Can you work these out from the model? Positions are in its coordinate system, mm. A direction names the side the tool comes from. Round coordinates to 2 decimals unless told otherwise and drop trailing zeros. Order: outer loops, then holes, each group sorted by start corner. A loop starts at its lowest first (then second) coordinate and runs counter-clockwise, first axis right, second up.
Q1. If we section it at D-D (y = 6.5): Please give me the cut outline in (x, z), plus the area to 3 significant figures.
Q2. If we section it at B-B (z = -5): Please give me the cut outline in (x, y).
Q3. We'd pull the mould along X, two halves only. Please class faces 1 (the face through (134.287, 1.662, 2.229)), 2 (the face through (1.713, 62.338, 2.229)), 3 (the face through (67, 32, 0)), 4 (the face through (67, 32, 2.5)): pulls with the +X half, pulls with the -X half, needs draft (parallel to the pull), parting line crosses it, or undercut.
Q4. For faces 5 (the face through (69.846, 53.951, -6.409)), 6 (the face through (1.662, 1.713, 2.229)), which set-ups out of +Z, -Z, +X, -X, +Y, -Y let a thin tool reach every point of the face, with its end or its side?
Q5. If we section it at A-A (x = 129.5): Please give me the cut outline in (y, z), plus the area to 3 significant figures.
Q6. If we section it at C-C (y = 57.5): Please give me the cut outline in (x, z), plus the area to 3 significant figures.
Q7. If I drill on line 1 (X direction, y = 57, z = -6.25); line 2 (X direction, y = 55, z = -8.5); line 3 (Z direction, x = 61, y = 21.5), over which ranges is the centre line in solid material (lowest first)?
Q8. Will these pins go through, and if not, where does the flat tip stop? P1, Ø1.5, axis at x = 71.5, y = 47.5, coming from the -Z side; P2, Ø1.5, axis at x = 36, z = -1, coming from the +Y side; P3, Ø4, axis at y = 12.5, z = -1, coming from the -X side.
from build123d import *

# Parameters (mm, degrees)
PAD_DEPTH       = 2.5
SKETCH002_R     = 4
PAD001_DEPTH    = 15
CHAMFER_SIZE    = 1
CHAMFER001_SIZE = 2


with BuildPart() as part:
    # Sketch → Pad (new body)
    with BuildSketch(Plane.XY):
        with BuildLine():
            Line((4, 0), (132, 0))
            ThreePointArc((132, 0), (134.828427, 1.171573), (136, 4))
            Line((136, 4), (136, 60))
            ThreePointArc((136, 60), (134.828427, 62.828427), (132, 64))
            Line((132, 64), (4, 64))
            ThreePointArc((4, 64), (1.171573, 62.828427), (0, 60))
            Line((0, 60), (0, 4))
            ThreePointArc((0, 4), (1.171573, 1.171573), (4, 0))
        make_face()
    extrude(amount=PAD_DEPTH)

    # Sketch002 → Pad001 (join)
    with BuildSketch(Plane.XY):
        with Locations((6.5, 6.5)):
            Circle(SKETCH002_R)
        with Locations((129.5, 6.5)):
            Circle(SKETCH002_R)
        with Locations((129.5, 57.5)):
            Circle(SKETCH002_R)
        with Locations((6.5, 57.5)):
            Circle(SKETCH002_R)
        with Locations((68, 57.5)):
            Circle(SKETCH002_R)
    extrude(amount=-PAD001_DEPTH)

    # Chamfer
    chamfer_edges = [part.edges().sort_by_distance(p)[0] for p in [
        (68, 0, 2.5),
        (134.828427, 1.171573, 2.5),
        (136, 32, 2.5),
        (134.828427, 62.828427, 2.5),
        (68, 64, 2.5),
        (1.171573, 62.828427, 2.5),
        (0, 32, 2.5),
        (1.171573, 1.171573, 2.5),
    ]]
    chamfer(chamfer_edges, length=CHAMFER_SIZE)

    # Chamfer001
    chamfer001_edges = [part.edges().sort_by_distance(p)[0] for p in [
        (2.5, 6.5, -15),
        (2.5, 57.5, -15),
        (64, 57.5, -15),
        (125.5, 57.5, -15),
        (125.5, 6.5, -15),
    ]]
    chamfer(chamfer001_edges, length=CHAMFER001_SIZE)


solid = part.part
Solution:
1. outline: (0, 0) - (2.5, 0) - (2.5, -13) - (4.5, -15) - (8.5, -15) - (10.5, -13) - (10.5, 0) - (125.5, 0) - (125.5, -13) - (127.5, -15) - (131.5, -15) - (133.5, -13) - (133.5, 0) - (136, 0) - (136, 1.5) - (135, 2.5) - (1, 2.5) - (0, 1.5) - close
1. area: 571 mm2
2. outline: circle Ø8 at (6.5, 6.5); circle Ø8 at (6.5, 57.5); circle Ø8 at (68, 57.5); circle Ø8 at (129.5, 6.5); circle Ø8 at (129.5, 57.5)
3. face 1: pulls with the +X half
3. face 2: pulls with the -X half
3. face 3: undercut
3. face 4: needs draft
4. face 5: -Z
4. face 6: +Z, -X, -Y
5. outline: (0, 0) - (2.5, 0) - (2.5, -13) - (4.5, -15) - (8.5, -15) - (10.5, -13) - (10.5, 0) - (53.5, 0) - (53.5, -13) - (55.5, -15) - (59.5, -15) - (61.5, -13) - (61.5, 0) - (64, 0) - (64, 1.5) - (63, 2.5) - (1, 2.5) - (0, 1.5) - close
5. area: 391 mm2
6. outline: (0, 0) - (2.5, 0) - (2.5, -13) - (4.5, -15) - (8.5, -15) - (10.5, -13) - (10.5, 0) - (64, 0) - (64, -13) - (66, -15) - (70, -15) - (72, -13) - (72, 0) - (125.5, 0) - (125.5, -13) - (127.5, -15) - (131.5, -15) - (133.5, -13) - (133.5, 0) - (136, 0) - (136, 1.5) - (135, 2.5) - (1, 2.5) - (0, 1.5) - close
6. area: 687 mm2
7. line 1: x = 2.53 to 10.47, 64.03 to 71.97, 125.53 to 133.47
7. line 2: x = 3.38 to 9.62, 64.88 to 71.12, 126.38 to 132.62
7. line 3: z = 0 to 2.5
8. P1: stops at z = 0
8. P2: passes through
8. P3: stops at x = 0
